Read the model definition and answer for the solid it produces. Units are mm, in the model's axes. A direction names the side the tool comes from. Coordinates: 2 decimals unless noted, no trailing zeros. Order: outer loops, then holes, each group sorted by start corner. A loop starts at its lowest first (then second) coordinate and runs counter-clockwise, first axis right, second up.
```python
from build123d import *

# Parameters (mm, degrees)
SKETCH1_W           = 42
SKETCH1_H           = 5.00807777
BOSS_EXTRUDE1_DEPTH = 18
SKETCH2_W           = 32.5
SKETCH2_H           = 12
CUT_EXTRUDE1_DEPTH  = 3
CUT_EXTRUDE2_REACH  = 29.821
SKETCH3_W           = 22.5
SKETCH3_H           = 12
CUT_EXTRUDE3_REACH  = 29.821
SKETCH4_W           = 5
SKETCH4_H           = 5


with BuildPart() as part:
    # Sketch1 → Boss-Extrude1 (new body)
    with BuildSketch(Plane.XY):
        with Locations((0, -2.504038885)):
            Rectangle(SKETCH1_W, SKETCH1_H)
    extrude(amount=BOSS_EXTRUDE1_DEPTH)

    # Sketch2 → Cut-Extrude1 (cut)
    with BuildSketch(Plane(origin=(0, 0, 0), x_dir=(1, 0, 0), z_dir=(0, 1, 0))):
        with Locations((0.75, -9)):
            Rectangle(SKETCH2_W, SKETCH2_H)
    extrude(amount=-CUT_EXTRUDE1_DEPTH, mode=Mode.SUBTRACT)

    # Sketch3 → Cut-Extrude2 (cut, up to next)
    with BuildSketch(Plane(origin=(0, -3, 0), x_dir=(1, 0, 0), z_dir=(0, 1, 0)), mode=Mode.PRIVATE) as cut_extrude2_sk1:
        with Locations((0.75, -9)):
            Rectangle(SKETCH3_W, SKETCH3_H)
    cut_extrude2_tool1 = extrude(cut_extrude2_sk1.sketch, amount=-CUT_EXTRUDE2_REACH, mode=Mode.PRIVATE) & part.part
    add(cut_extrude2_tool1.solids().sort_by_distance((0.75, -3, 9))[0], mode=Mode.SUBTRACT)

    # Sketch4 → Cut-Extrude3 (cut, up to next)
    with BuildSketch(Plane(origin=(0, -3, 0), x_dir=(1, 0, 0), z_dir=(0, 1, 0)), mode=Mode.PRIVATE) as cut_extrude3_sk1:
        with Locations((14.5, -9)):
            Rectangle(SKETCH4_W, SKETCH4_H)
    cut_extrude3_tool1 = extrude(cut_extrude3_sk1.sketch, amount=-CUT_EXTRUDE3_REACH, mode=Mode.PRIVATE) & part.part
    add(cut_extrude3_tool1.solids().sort_by_distance((14.5, -3, 9))[0], mode=Mode.SUBTRACT)


solid = part.part
```
1) A cutting plane is placed at D-D, the plane z = 13.25. Determine the outline of the cut face in (x, y).
A:
outline: (-21, -5.01) - (-10.5, -5.01) - (-10.5, -3) - (-15.5, -3) - (-15.5, 0) - (-21, 0) - close; (12, -5.01) - (21, -5.01) - (21, 0) - (17, 0) - (17, -3) - (12, -3) - close
2) Flat-ended cylindrical pins translate along their axes: pin 1 Ø2 at (x, z) = (8.5, 12.5) entering from +Y; pin 2 Ø1.5 at (x, z) = (-13.5, 12) entering from +Y. Find the tip coordinate at first contact, or state that the pin passes through.
A:
pin 1: passes through
pin 2: stops at y = -3
3) Determine the mould class of faces 4 (the flat face through (0, -2, 0)), 5 (the flat face through (0, -2, 18)), 6 (the flat face through (14, -4, 11.5)), 7 (the flat face through (0, -5.008, 1)) for opening direction Z: pulls with the +Z half, pulls with the -Z half, needs draft (parallel to the pull), parting line crosses it, or undercut.
A:
face 4: pulls with the -Z half
face 5: pulls with the +Z half
face 6: undercut
face 7: needs draft
4) Which of the six approach directions +Z, -Z, +X, -X, +Y, -Y give full straight-line access (tool end or side, diameter ignored) to faces 1 (the flat face through (1, -2, 3)), 2 (the flat face through (12, -4, 5)), 3 (the flat face through (0, 0, 1))?
A:
face 1: +Y
face 2: +Y, -Y
face 3: +Z, -Z, +X, -X, +Y
5) A cutting plane is placed at A-A, the plane z = 8. Determine the outline of the cut face in (x, y).
A:
outline: (-21, -5.01) - (-10.5, -5.01) - (-10.5, -3) - (-15.5, -3) - (-15.5, 0) - (-21, 0) - close; (17, -5.01) - (21, -5.01) - (21, 0) - (17, 0) - close
6) A cutting plane is placed at B-B, the plane x = -7.5. Determine the outline of the cut face in (y, z), and give its area (3 significant figures).
A:
outline: (-5.01, 0) - (0, 0) - (0, 3) - (-5.01, 3) - close; (-5.01, 15) - (0, 15) - (0, 18) - (-5.01, 18) - close
area: 30.0 mm2
7) A cutting plane is placed at C-C, the plane y = -3.9. Determine the outline of the cut face in (x, z).
A:
outline: (-21, 0) - (21, 0) - (21, 18) - (-21, 18) - close; hole (-10.5, 3) - (12, 3) - (12, 6.5) - (17, 6.5) - (17, 11.5) - (12, 11.5) - (12, 15) - (-10.5, 15) - close
8) Straight lines are drawn through the part: line 1 (X direction, y = -3.5, z = 9.5); line 2 (X direction, y = -1.95, z = 12.25); line 3 (Z direction, x = -3.5, y = -2.35). For each, find the intervals that lie inside material, in ascending order.
A:
line 1: x = -21 to -10.5, 17 to 21
line 2: x = -21 to -15.5, 17 to 21
line 3: z = 0 to 3, 15 to 18
